Read the model definition and answer for the solid it produces. Units are mm, in the model's axes. Coordinates: 2 decimals unless noted, no trailing zeros. Order: outer loops, then holes, each group sorted by start corner. A loop starts at its lowest first (then second) coordinate and runs counter-clockwise, first axis right, second up. Notation, with made-up numbers: (-30, 8) -> (4, 8) arc R10 ccw to (4, 15) -> close; hole circle Ø6 at (26, -33). An arc over 180 degrees is marked (long way). Answer in a Markdown table with one row per item.
Autodesk Inventor part; units mm, degrees
ref_plane "YZ Plane" through (0, 0, 0) normal (1, 0, 0) x (0, 1, 0)
ref_plane "XZ Plane" through (0, 0, 0) normal (0, 1, 0) x (-1, 0, 0)
ref_plane "XY Plane" through (0, 0, 0) normal (0, 0, 1) x (1, 0, 0)
sketch "Sketch1" plane through (0, 0, 0) normal (0, 1, 0) x (-1, 0, 0)
  line L0 (-168.91, 205.74) -> (168.91, 205.74)
  line L1 (168.91, 205.74) -> (168.91, -205.74)
  line L2 (168.91, -205.74) -> (-168.91, -205.74)
  line L3 (-168.91, -205.74) -> (-168.91, 205.74)
  line L4 (-168.91, 205.74) -> (168.91, -205.74) construction
  line L5 (168.91, 205.74) -> (-168.91, -205.74) construction
  point P0 (0, 0)
  dimension "d0" = 411.48
  dimension "d1" = 337.82
extrude "Extrusion1" add sketch "Sketch1" along normal blind 65.024
sketch "Sketch2" plane through (168.91, 0, 205.74) normal (1, 0, 0) x (0, 0, -1)
  line L0 (102.87, 65.024) -> (308.61, 65.024)
  line L1 (411.48, 0) -> (411.48, 23.876)
  line L2 (308.61, 65.024) -> (411.48, 23.876)
  line L3 (411.48, 0) -> (411.48, 65.024)
  line L4 (308.61, 65.024) -> (411.48, 65.024)
  line L5 (411.48, 65.024) -> (411.48, 23.876)
  line L6 (102.87, 65.024) -> (0, 23.876)
  line L7 (0, 23.876) -> (0, 65.024)
  line L8 (0, 65.024) -> (102.87, 65.024)
  line L9 (411.48, 0) -> (0, 0)
  point P0 (205.74, 0)
  point P1 (205.74, 65.024)
  point P2 (205.74, 65.024)
  dimension "d4" = 205.74
  dimension "d5" = 23.876
  dimension "d6" = 23.876
extrude "Extrusion2" cut sketch "Sketch2" against normal blind 387.2865
sketch "Sketch3" plane through (0, 65.024, 0) normal (0, 1, 0) x (1, 0, 0)
  line L0 (60.325, -60.325) -> (-60.325, -60.325)
  line L1 (-60.325, -60.325) -> (-60.325, 60.325)
  line L2 (-60.325, 60.325) -> (60.325, 60.325)
  line L3 (60.325, 60.325) -> (60.325, -60.325)
  line L4 (60.325, -60.325) -> (-60.325, 60.325) construction
  line L5 (-60.325, -60.325) -> (60.325, 60.325) construction
  point P0 (0, 0)
  dimension "d9" = 120.65
  dimension "d10" = 120.65
extrude "Extrusion3" cut sketch "Sketch3" against normal blind 7.1437
sketch "Sketch4" plane through (0, 57.8803, 0) normal (0, 1, 0) x (1, 0, 0)
  circle A0 centre (-50.0276, 50.2457) radius 1.5875
  circle A1 centre (49.9724, 50.2457) radius 1.5875
  circle A2 centre (49.9724, -49.7543) radius 1.5875
  circle A3 centre (-50.0276, -49.7543) radius 1.5875
  point P0 (0, 0)
  dimension "d13" = 3.175
  dimension "d14" = 3.175
  dimension "d15" = 3.175
  dimension "d16" = 3.175
  dimension "d17" = 100
  dimension "d18" = 100
  dimension "d19" = 100
extrude "Extrusion4" cut sketch "Sketch4" against normal blind 7.62
properties part number "monitor (for assembly)"
Q1. The part is cut by section C-C (x = -147.5). Write down the section's boundary in (y, z), then the cut area to 3 significant figures.
Outcome:
| item | result |
|---|---|
| outline | (0, -205.74) -> (23.88, -205.74) -> (65.02, -102.87) -> (65.02, 102.87) -> (23.88, 205.74) -> (0, 205.74) -> close |
| area | 22,500 mm² |
Q2. The part is cut by section A-A (z = 28). Write down the section's boundary in (x, y) (3 decimals), then the cut area to 3 significant figures.
Outcome:
| item | result |
|---|---|
| outline | (-168.91, 0) -> (168.91, 0) -> (168.91, 65.024) -> (60.325, 65.024) -> (60.325, 57.88) -> (-60.325, 57.88) -> (-60.325, 65.024) -> (-168.91, 65.024) -> close |
| area | 21,100 mm² |
Q3. The part is cut by section D-D (z = 133.5). Write down the section's boundary in (x, y).
Outcome:
| item | result |
|---|---|
| outline | (-168.91, 0) -> (168.91, 0) -> (168.91, 52.77) -> (-168.91, 52.77) -> close |
Q4. Given pin 1 (1.6 mm diameter, centred on x = -49.5, z = -51, fed in from +Y); pin 2 (2.5 mm diameter, centred on x = -50.03, z = -50.25, fed in from +Y), each flat-ended and moving along its own axis, determine where each tip first touches the part or whether it passes through.
Outcome:
| item | result |
|---|---|
| pin 1 | y = 57.88 |
| pin 2 | y = 50.26 |
Q5. Consider line 1 (Y direction, x = 16, z = -16.5); line 2 (Z direction, x = -46.5, y = 45). Determine where each line is inside the solid, lowest interval first.
Outcome:
| item | result |
|---|---|
| line 1 | 0 to 57.88 |
| line 2 | -152.93 to 152.93 |
Q6. For a pull along Z with two mould halves and no side action, classify faces 1 (the face through (168.91, 25, -3)), 2 (the face through (-2, 12, -205.74)), 3 (the face through (-1, 57.88, -1)) as pulls with the +Z half, pulls with the -Z half, needs draft (parallel to the pull), parting line crosses it, or undercut.
Outcome:
| item | result |
|---|---|
| face 1 | needs draft |
| face 2 | pulls with the -Z half |
| face 3 | undercut |
Q7. The part is cut by section B-B (y = 45.5). Write down the section's boundary in (x, z).
Outcome:
| item | result |
|---|---|
| outline | (-168.91, -151.68) -> (168.91, -151.68) -> (168.91, 151.68) -> (-168.91, 151.68) -> close |
